Source: CAD feature listing. Evaluate the final solid. Frame: model axes, mm. A direction names the side the tool comes from. Round coordinates to 2 decimals unless told otherwise and drop trailing zeros. Write each loop counter-clockwise with the first axis right and the second up, starting at its lowest first coordinate (ties: lowest second). Pieces come first, ordered by that corner, then holes. Notation, with made-up numbers: M 45.5,-34 L 56.5,-34 A21 ccw 56.5,-16 Z; hole C 59.25,76.25 d11. An arc over 180 degrees is marked long. Answer in a Markdown table with one row per item.
from build123d import *

# Parameters (mm, degrees)
F1_DEPTH    = 6
F2_W        = 10
F2_H        = 30
F3_DEPTH    = 6
F4_R        = 1.5
F5_DEPTH    = 34.001
F6_T1_DEPTH = 242.8543856465


# Not quite as in the source:
# - a fillet or chamfer that OpenCascade refuses, or shapes differently, is made with other operations: its cross-section is extruded or revolved along the edge and cut away or added


with BuildPart() as f1:
    # F0 (on Top) → F1 (new body)
    with BuildSketch(Plane.XY):
        Polygon((7, -150), (17, -150), (17, 150), (-17, 150), (-17, -150), (-7, -150), (-7, 10), (-5, 10), (-5, -120), (5, -120), (5, 10), (7, 10), align=None)
    extrude(amount=F1_DEPTH)

    # F2 (on face) → F3 (join)
    with BuildSketch(Plane.XY.offset(6)):
        with Locations((-12, -135)):
            Rectangle(F2_W, F2_H)
        with Locations((12, -135)):
            Rectangle(F2_W, F2_H)
    extrude(amount=F3_DEPTH)

    # F4 (on face) → F5 (cut, through all)
    with BuildSketch(Plane(origin=(-17, 0, 0), x_dir=(0, -1, 0), z_dir=(-1, 0, 0))):
        with Locations((136.3040655851, 6)):
            Circle(F4_R)
    extrude(amount=-F5_DEPTH, mode=Mode.SUBTRACT)

    # F6: fillet of radius 50 on 1 edges, made by hand

    # F6_s2 → F6_t1 (cut)
    with BuildSketch(Plane.XY.offset(-118.4271928233)):
        with BuildLine():
            ThreePointArc((17, 102.6291228707), (7.6201920232, 131.7838823449), (-17, 150))
            Line((-17, 150), (17, 150))
            Line((17, 150), (17, 102.6291228707))
        make_face()
    extrude(amount=F6_T1_DEPTH, mode=Mode.SUBTRACT)


solid = f1.part
Q1. Section D-D (y = 99). Return loops of the section in (x, z), and give its area (3 significant figures).
Solutions:
| item | result |
|---|---|
| outline | M -17,0 L 17,0 L 17,6 L -17,6 Z |
| area | 204 mm2 |
Q2. Access query for faces 1 (the flat face through (12, -120, 9)), 2 (the cylindrical face through (7.87, 131.43, 2.96)), 3 (the flat face through (0, -120, 3)). Directions: +Z, -Z, +X, -X, +Y, -Y. A direction counts if a zero-diameter tool reaches every point of the face in a straight line with its end or side. Return the directions, or none.
Solutions:
| item | result |
|---|---|
| face 1 | +Z, +X, -X, +Y |
| face 2 | +Z, -Z, +X, +Y |
| face 3 | +Z, -Z, -Y |
Q3. Section A-A (y = -10). Return loops of the section in (x, z).
Solutions:
| item | result |
|---|---|
| outline | M -17,0 L -7,0 L -7,6 L -17,6 Z; M -5,0 L 5,0 L 5,6 L -5,6 Z; M 7,0 L 17,0 L 17,6 L 7,6 Z |
Q4. Contact query for flat-ended pins moving along their axis: pin 1 Ø4 at (x, z) = (-0.5, 8.5) entering from +Y; pin 2 Ø1.8 at (x, z) = (12, 9.5) entering from +Y; pin 3 Ø1 at (x, z) = (-6, 4.5) entering from -Y; pin 4 Ø5 at (x, z) = (-12.5, 8) entering from +Y. Output: stop coordinate, or through.
Solutions:
| item | result |
|---|---|
| pin 1 | passes through |
| pin 2 | stops at y = -120 |
| pin 3 | stops at y = 10 |
| pin 4 | stops at y = 148.88 |
Q5. Section B-B (x = -10). Return loops of the section in (y, z), and give its area (3 significant figures).
Solutions:
| item | result |
|---|---|
| outline | M -150,0 L 147.03,0 L 147.03,6 L -120,6 L -120,12 L -150,12 Z; hole C -136.3,6 d3 |
| area | 1,960 mm2 |
Q6. Material intervals for probe 1 along X at (y, z) = (-119.5, 4); probe 2 along X at (y, z) = (-121.5, 9); probe 3 along Z at (x, y) = (-14.5, 35), sorted ascending.
Solutions:
| item | result |
|---|---|
| probe 1 | x = -17 to -7, -5 to 5, 7 to 17 |
| probe 2 | x = -17 to -7, 7 to 17 |
| probe 3 | z = 0 to 6 |
Q7. Section C-C (z = 2). Return loops of the section in (x, y).
Solutions:
| item | result |
|---|---|
| outline | M -17,-150 L -7,-150 L -7,10 L -5,10 L -5,-120 L 5,-120 L 5,10 L 7,10 L 7,-150 L 17,-150 L 17,102.63 A50 ccw -17,150 Z |
